```python
from build123d import *

# Parameters (mm, degrees)
F0_W      = 43
F0_H      = 31
F1_DEPTH  = 16
F2_T      = -2
F3_R      = 3.25
F4_DEPTH  = 16.001
F5_R      = 3
F6_DEPTH  = 7.6
F7_W      = 5
F7_H      = 5
F8_DEPTH  = 14
F9_W      = 5
F9_H      = 5
F10_DEPTH = 14
F12_R     = 1
F13_DEPTH = 10
F14_R     = 4.5
F15_DEPTH = 1


with BuildPart() as f1:
    # F0 (on Front) → F1 (new body)
    with BuildSketch(Plane.XZ):
        Rectangle(F0_W, F0_H)
    extrude(amount=F1_DEPTH)

    # F2
    f2_openings = [f1.faces().sort_by_distance(p)[0] for p in [
        (0, 0, 0),
    ]]
    offset(amount=F2_T, openings=f2_openings)

    # F3 (on face) → F4 (cut, through all)
    with BuildSketch(Plane.XZ.offset(16)):
        with Locations((0, 8)):
            Circle(F3_R)
        with Locations((0, -8)):
            Circle(F3_R)
    extrude(amount=-F4_DEPTH, mode=Mode.SUBTRACT)

    # F5 (on face) → F6 (cut)
    with BuildSketch(Plane.YZ.offset(21.5)):
        with Locations((-6, 0)):
            Circle(F5_R)
    extrude(amount=-F6_DEPTH, mode=Mode.SUBTRACT)

    # F7 (on face) → F8 (join, through all)
    with BuildSketch(Plane(origin=(0, 0, 0), x_dir=(-1, 0, 0), z_dir=(0, 1, 0))):
        with Locations((17, 11)):
            Rectangle(F7_W, F7_H)
    extrude(amount=-F8_DEPTH)


with BuildPart() as f10:
    # F9 (on face) → F10 (new body, through all)
    with BuildSketch(Plane(origin=(0, 0, 0), x_dir=(-1, 0, 0), z_dir=(0, 1, 0))):
        with Locations((17, -11)):
            Rectangle(F9_W, F9_H)
        with Locations((-17, -11)):
            Rectangle(F9_W, F9_H)
        with Locations((-17, 11)):
            Rectangle(F9_W, F9_H)
    extrude(amount=-F10_DEPTH)


with BuildPart() as f1_1:
    add(f1.part)

    # F11: union F10
    add(f10.part)

    # F12 (on face) → F13 (cut)
    with BuildSketch(Plane(origin=(0, 0, 0), x_dir=(-1, 0, 0), z_dir=(0, 1, 0))):
        with Locations((18, 12)):
            Circle(F12_R)
        with Locations((18, -12)):
            Circle(F12_R)
        with Locations((-18, 12)):
            Circle(F12_R)
        with Locations((-18, -12)):
            Circle(F12_R)
    extrude(amount=-F13_DEPTH, mode=Mode.SUBTRACT)

    # F14 (on face) → F15 (cut)
    with BuildSketch(Plane(origin=(0, -14, 0), x_dir=(-1, 0, 0), z_dir=(0, 1, 0))):
        with Locations((-14, 0)):
            Circle(F14_R)
        with Locations((14, 0)):
            Circle(F14_R)
    extrude(amount=-F15_DEPTH, mode=Mode.SUBTRACT)


solid = f1_1.part
```
Part model, mm, in its own coordinate system. A direction names the side the tool comes from. Round coordinates to 2 decimals unless told otherwise and drop trailing zeros. Loops run counter-clockwise (first coordinate to the right, second up) from the corner with the lowest first, then second, coordinate; pieces in that order, holes last.
1. Slice it at C-C (y = -0.75). Give the cut face in (x, z), and give its area (3 significant figures).
Solutions:
outline: (-21.5, -15.5) - (21.5, -15.5) - (21.5, 15.5) - (-21.5, 15.5) - close; hole (-19.5, -8.5) - (-14.5, -8.5) - (-14.5, -13.5) - (14.5, -13.5) - (14.5, -8.5) - (19.5, -8.5) - (19.5, 8.5) - (14.5, 8.5) - (14.5, 13.5) - (-14.5, 13.5) - (-14.5, 8.5) - (-19.5, 8.5) - close; hole circle Ø2 at (-18, -12); hole circle Ø2 at (-18, 12); hole circle Ø2 at (18, -12); hole circle Ø2 at (18, 12)
area: 367 mm2
2. Flat gauge pin, fed straight in: pin 1 (7 mm diameter, centred on x = -12, z = -2, fed in from +Y). Where does the tip first touch, or does it go through?
Solutions:
pin 1: stops at y = -14
3. Slice it at D-D (x = 14). Give the cut face in (y, z).
Solutions:
outline: (-16, -15.5) - (0, -15.5) - (0, -13.5) - (-14, -13.5) - (-14, -4.5) - (-15, -4.5) - (-15, 4.5) - (-14, 4.5) - (-14, 13.5) - (0, 13.5) - (0, 15.5) - (-16, 15.5) - close
4. Two-plate mould, pull along Z, no slides. Class faces 1 (the face through (-21.5, -8, 0)), 2 (the face through (-18, -10, 12)), 3 (the face through (0, -8, 15.5)): pulls with the +Z half, pulls with the -Z half, needs draft (parallel to the pull), parting line crosses it, or undercut.
Solutions:
face 1: needs draft
face 2: undercut
face 3: pulls with the +Z half
5. Drill centre lines: line 1 along Z through (x, y) = (0, -15.1); line 2 along Z through (x, y) = (-18, -7.25); line 3 along Z through (x, y) = (13, -11). Where is each one in solid material? Low to high.
Solutions:
line 1: z = -15.5 to -11.25, -4.75 to 4.75, 11.25 to 15.5
line 2: z = -15.5 to -13, -11 to -8.5, 8.5 to 11, 13 to 15.5
line 3: z = -15.5 to -13.5, 13.5 to 15.5
6. 3-axis set-ups, long thin cutter, end or side, ignore diameter. For faces 4 (the face through (-17, -7, -8.5)), 5 (the face through (-0.423, -15.014, -4.778)), 6 (the face through (20.51, -3.14, 0.9)): which of +Z, -Z, +X, -X, +Y, -Y reach the whole face in a straight line?
Solutions:
face 4: +Y
face 5: +Y, -Y
face 6: +X
7. Slice it at B-B (x = 0). Give the cut face in (y, z).
Solutions:
outline: (-16, -15.5) - (0, -15.5) - (0, -13.5) - (-14, -13.5) - (-14, -11.25) - (-16, -11.25) - close; (-16, -4.75) - (-14, -4.75) - (-14, 4.75) - (-16, 4.75) - close; (-16, 11.25) - (-14, 11.25) - (-14, 13.5) - (0, 13.5) - (0, 15.5) - (-16, 15.5) - close
8. Slice it at A-A (z = 0). Give the cut face in (x, y), and give its area (3 significant figures).
Solutions:
outline: (-21.5, -16) - (21.5, -16) - (21.5, -9) - (19.5, -9) - (19.5, -14) - (18.5, -14) - (18.5, -15) - (9.5, -15) - (9.5, -14) - (-9.5, -14) - (-9.5, -15) - (-18.5, -15) - (-18.5, -14) - (-19.5, -14) - (-19.5, 0) - (-21.5, 0) - close; (19.5, -3) - (21.5, -3) - (21.5, 0) - (19.5, 0) - close
area: 112 mm2
